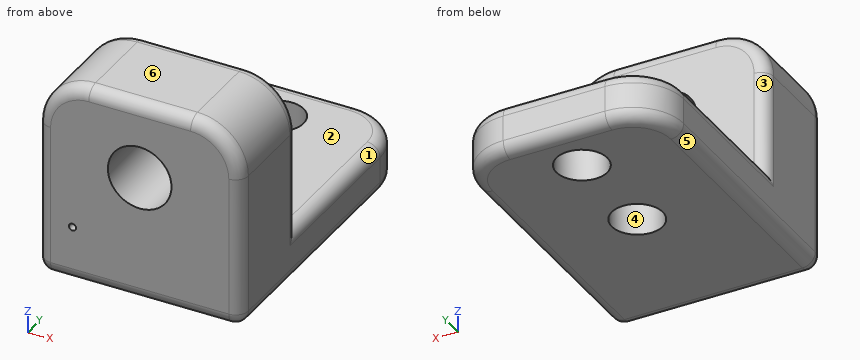
Autodesk Inventor part; units mm, degrees
ref_plane "YZ Plane" through (0, 0, 0) normal (1, 0, 0) x (0, 1, 0)
ref_plane "XZ Plane" through (0, 0, 0) normal (0, 1, 0) x (-1, 0, 0)
ref_plane "XY Plane" through (0, 0, 0) normal (0, 0, 1) x (1, 0, 0)
sketch "Sketch1" plane through (0, 0, 0) normal (0, 0, 1) x (1, 0, 0)
  line L0 (0, 0) -> (25.4, 0)
  line L1 (25.4, 0) -> (25.4, 38.1)
  line L2 (25.4, 38.1) -> (0, 38.1)
  line L3 (0, 38.1) -> (0, 0)
  dimension "d0" = 38.1
  dimension "d1" = 25.4
extrude "Extrusion1" add sketch "Sketch1" along normal blind 25.4
sketch "Sketch4" plane through (25.4, 0, 0) normal (1, 0, 0) x (0, 0, -1)
  line L0 (0, 0) -> (-25.4, 0)
  line L1 (0, 0) -> (0, 38.1)
  line L2 (-25.4, 38.1) -> (-6.35, 38.1)
  line L3 (-6.35, 38.1) -> (-6.35, 12.7)
  line L4 (-6.35, 12.7) -> (-25.4, 12.7)
  line L5 (-25.4, 12.7) -> (-25.4, 38.1)
  dimension "d23" = 6.35
  dimension "d24" = 12.7
extrude "Extrusion4" cut sketch "Sketch4" against normal through all
sketch "Sketch3" plane through (0, 0, 0) normal (0, 0, -1) x (-1, 0, 0)
  line L0 (-25.4, 38.1) -> (0, 38.1)
  line L1 (-25.4, 0) -> (-25.4, 38.1)
  circle A0 centre (-12.7, 31.75) radius 3.175
  circle A1 centre (-12.7, 19.05) radius 3.175
  dimension "d11" = 6.35
  dimension "d12" = 6.35
  dimension "d13" = 12.7
  dimension "d14" = 12.7
  dimension "d22" = 12.7
extrude "Extrusion3" cut sketch "Sketch3" against normal through all
sketch "Sketch5" plane through (0, 0, 0) normal (0, -1, 0) x (1, 0, 0)
  line L0 (25.4, 25.4) -> (0, 25.4)
  line L1 (25.4, 0) -> (25.4, 25.4)
  circle A0 centre (12.7, 15.875) radius 3.9688
  dimension "d27" = 9.525
  dimension "d28" = 7.9375
  dimension "d29" = 12.7
extrude "Extrusion5" cut sketch "Sketch5" against normal up to next
fillet "Fillet4" radius 1.5875 13 edges at (12.7, 38.1, 6.35) (12.7, 38.1, 0) (0, 25.4, 6.35) (0, 19.05, 0) (25.4, 25.4, 6.35) (25.4, 19.05, 0) (12.7, 0, 0) (25.4, 0, 12.7) (0, 0, 12.7) (25.4, 12.7, 15.875) (0, 12.7, 15.875) (12.7, 12.7, 25.4) (12.7, 0, 25.4)
fillet "Fillet5" radius 6.35 12 edges at (0.465, 12.235, 24.935) (0.465, 0.465, 24.935) (0, 6.35, 25.4) (24.935, 0.465, 24.935) (24.935, 12.235, 24.935) (25.4, 6.35, 25.4) (0.465, 37.635, 5.885) (0.465, 37.635, 0.465) (0, 38.1, 3.175) (24.935, 37.635, 5.885) (24.935, 37.635, 0.465) (25.4, 38.1, 3.175)
sketch "Sketch6" plane through (1.5875, 0, 1.5875) normal (0, -1, 0) x (1, 0, 0)
  circle A0 centre (2.7307, 5.3937) radius 0.4473
  point P0 (-1.5875, -1.5875)
extrude "Extrusion6" cut sketch "Sketch6" against normal blind 2.54
properties part number "MainLiftBlock" material "Aluminum-6061"
Could you check a few things on this model? Use its own coordinates, in mm. Face numbers are marked on the shaded views. A direction names the side the tool comes from. Give positions to 0.01 mm unless a question says otherwise; leave off trailing zeros. One line per item, written item: value. Start each with the question number.
Item 1: I'm going to push flat-ended pins straight in: pin 1 (7.5 mm diameter, centred on x = 12.7, y = 31.75, fed in from -Z); pin 2 (12 mm diameter, centred on x = 5, y = 18, fed in from +Z); pin 3 (10.5 mm diameter, centred on x = 12.7, z = 15.875, fed in from +Y). Where does each tip first touch, or does it pass through?
Item 2: If we mould it in two halves opening along X, with no side actions, what happens to the marked faces 4, 5 and 6? For each: +X half, -X half, draft (parallel to the pull), parting line (faces both ways), or undercut.
Item 3: Please list where these lines run through material, in increasing order: line 1 (Y direction, x = 12.7, z = 1.5) (3 decimals); line 2 (Y direction, x = 10.5, z = 5.25); line 3 (Z direction, x = 12.7, y = 4.5). Write a range as from..to.
Item 4: Which directions (+Z, -Z, +X, -X, +Y, -Y) give clear straight access to the entire face, cutting with the end or side of a thin tool? Please do the marked faces 1, 2 and 3.
Item 5: Imagine slicing it at C-C, the plane x = 12.7. Give the number of separate pieces and of enclosed holes in the cut face, and give its area (3 significant figures).
Geometry says:
1. pin 1: z = 0
1. pin 2: z = 25.07
1. pin 3: y = 12.7
2. face 4: undercut
2. face 5: -X half
2. face 6: draft
3. line 1: 0.002..15.875, 22.225..28.575, 34.925..38.098
3. line 2: 0..16.76, 21.34..29.46, 34.04..38.02
3. line 3: 0..11.91, 19.84..25.4
4. face 1: +Z, +X, +Y
4. face 2: +Z, +X, -X, +Y
4. face 3: +Z, -X, +Y
5. separate pieces: 4
5. enclosed holes: 0
5. area: 300 mm^2
